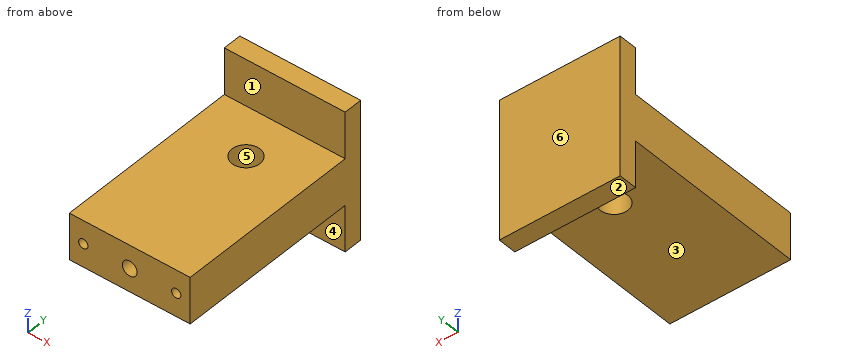
```python
from build123d import *

# Parameters (mm, degrees)
SKETCH1_W                = 13
SKETCH1_H                = 5
BOSS_EXTRUDE1_DEPTH      = 20
M2_TAPPED_HOLE1_D        = 1.6
M2_TAPPED_HOLE1_DEPTH    = 5.2
M2_TAPPED_HOLE1_TIP      = 0.480688495
F_3_0_3_DIAMETER_HOLE1_D = 3
SKETCH7_W                = 13
SKETCH7_H                = 15
BOSS_EXTRUDE2_DEPTH      = 2


with BuildPart() as part:
    # Sketch1 → Boss-Extrude1 (new body)
    with BuildSketch(Plane(origin=(0, 0, 0), x_dir=(1, 0, 0), z_dir=(0, 1, 0))):
        Rectangle(SKETCH1_W, SKETCH1_H)
    extrude(amount=BOSS_EXTRUDE1_DEPTH)

    # M2 Tapped Hole1
    with Locations(Plane(origin=(0, 0, 0), x_dir=(0, 0, -1), z_dir=(0, -1, 0))):
        with Locations((0, 0)):
            Hole(M2_TAPPED_HOLE1_D / 2, depth=M2_TAPPED_HOLE1_DEPTH)
            with Locations((0, 0, -(M2_TAPPED_HOLE1_DEPTH + M2_TAPPED_HOLE1_TIP / 2))):  # 118° drill point
                Cone(0, M2_TAPPED_HOLE1_D / 2, M2_TAPPED_HOLE1_TIP, mode=Mode.SUBTRACT)

    # Sketch4 → Ø1.0mm Dowel Hole1 (revolve, cut)
    with BuildSketch(Plane(origin=(-5, 0, 0), x_dir=(0, 0, -1), z_dir=(1, 0, 0))):
        Polygon((0, 0), (0, 4.30043031), (0.5, 4), (0.5, 0), align=None)
    f_1_0mm_dowel_hole1 = revolve(axis=Axis((-5, -6.35, 0), (0, 1, 0)), mode=Mode.SUBTRACT)

    # Mirror1: Ø1.0mm Dowel Hole1 across plane
    add(f_1_0mm_dowel_hole1.mirror(Plane(origin=(0, 0, 0), x_dir=(0, 0, 1), z_dir=(1, 0, 0))), mode=Mode.SUBTRACT)

    # Ø3.0 (3) Diameter Hole1 (through all)
    with Locations(Plane(origin=(0, 15, 2.5), x_dir=(1, 0, 0), z_dir=(0, 0, 1))):
        with Locations((0, 0)):
            Hole(F_3_0_3_DIAMETER_HOLE1_D / 2)

    # Sketch7 → Boss-Extrude2 (add)
    with BuildSketch(Plane(origin=(0, 20, 0), x_dir=(1, 0, 0), z_dir=(0, 1, 0))):
        Rectangle(SKETCH7_W, SKETCH7_H)
    extrude(amount=BOSS_EXTRUDE2_DEPTH)


solid = part.part
```
The listing builds one solid part. Answer for the finished solid, in the listing's coordinates (mm). Face numbers are marked on the shaded views. A direction names the side the tool comes from. Round coordinates to 2 decimals unless told otherwise and drop trailing zeros. Write each loop counter-clockwise with the first axis right and the second up, starting at its lowest first coordinate (ties: lowest second). Pieces come first, ordered by that corner, then holes. Notation, with made-up numbers: (66, 87.5) -> (70, 87.5) arc R35 ccw to (70, 121.5) -> close; hole circle Ø3 at (77, 86). An arc over 180 degrees is marked (long way). Answer as a JSON object with one key per item and string values. Group by question number.
Q1. Determine the mould class of the marked faces 3, 4, 5 and 6 for opening direction Y: pulls with the +Y half, pulls with the -Y half, needs draft (parallel to the pull), parting line crosses it, or undercut.
Q2. Section A-A (y = 15) is taken. Write down the section's boundary in (x, z).
Q3. Straight lines are drawn through the part: line 1 along Z through (x, y) = (-5, 2.7); line 2 along X through (y, z) = (3.2, 0); line 3 along Z through (x, y) = (-5, 16). For each, find the intervals that lie inside material, in ascending order.
Q4. Section C-C (y = 9.75) is taken. Write down the section's boundary in (x, z).
Q5. Which of the six approach directions +Z, -Z, +X, -X, +Y, -Y give full straight-line access (tool end or side, diameter ignored) to the marked faces 1 and 2?
Q6. Each of these flat-tipped pins is pushed along its axis until it touches: pin 1 Ø1.5 at (x, y) = (-2.5, 8) entering from -Z; pin 2 Ø2.5 at (x, z) = (-2, 4.5) entering from -Y; pin 3 Ø3 at (x, y) = (3.5, 12.5) entering from +Z. Where does it stop, or does it pass through?
Q7. Section B-B (z = -3.75) is taken. Write down the section's boundary in (x, y).
Check values:
{
 "1": {"face 3": "needs draft", "face 4": "pulls with the -Y half", "face 5": "undercut", "face 6": "pulls with the +Y half"},
 "2": {"outline": "(-6.5, -2.5) -> (-1.5, -2.5) -> (-1.5, 2.5) -> (-6.5, 2.5) -> close; (1.5, -2.5) -> (6.5, -2.5) -> (6.5, 2.5) -> (1.5, 2.5) -> close"},
 "3": {"line 1": "-2.5 to -0.5, 0.5 to 2.5", "line 2": "-6.5 to -5.5, -4.5 to -0.8, 0.8 to 4.5, 5.5 to 6.5", "line 3": "-2.5 to 2.5"},
 "4": {"outline": "(-6.5, -2.5) -> (6.5, -2.5) -> (6.5, 2.5) -> (-6.5, 2.5) -> close"},
 "5": {"face 1": "+Z, +X, -X, -Y", "face 2": "-Z, +X, -X, +Y, -Y"},
 "6": {"pin 1": "z = -2.5", "pin 2": "y = 20", "pin 3": "z = 2.5"},
 "7": {"outline": "(-6.5, 20) -> (6.5, 20) -> (6.5, 22) -> (-6.5, 22) -> close"}
}
